Work out the finished part from the listing and answer in its coordinate system (mm). A direction names the side the tool comes from. Give positions to 0.01 mm unless a question says otherwise; leave off trailing zeros. Order: outer loops, then holes, each group sorted by start corner. A loop starts at its lowest first (then second) coordinate and runs counter-clockwise, first axis right, second up. Notation, with made-up numbers: (-31.5, 15) - (26.5, 15) arc R23 ccw to (26.5, 27) - close; hole circle Ø1 at (-12, 45.25). An arc over 180 degrees is marked (long way). Put each result on its own line as item: value.
```python
from build123d import *

# Parameters (mm, degrees)
F1_DEPTH = 25.4


with BuildPart() as f1:
    # F0 (on Front) → F1 (new body)
    with BuildSketch(Plane.XZ):
        with BuildLine():
            Line((5.7565809201, 24.7419614515), (-18.5488766964, 17.3563260415))
            Line((-18.5488766964, 17.3563260415), (-24.3054576165, -7.38563541))
            Line((-24.3054576165, -7.38563541), (-5.7565809201, -24.7419614515))
            Line((-5.7565809201, -24.7419614515), (18.5488766964, -17.3563260415))
            Line((18.5488766964, -17.3563260415), (9.9212024357, -6.0961798708))
            ThreePointArc((9.9212024357, -6.0961798708), (-11.27855426, -2.8961837982), (5.7565809201, 10.1220276081))
            Line((5.7565809201, 10.1220276081), (5.7565809201, 24.7419614515))
        make_face()
        with BuildLine():
            ThreePointArc((11.6444693648, 0), (10.0654358316, 5.8549695395), (5.7565809201, 10.1220276081))
            Line((5.7565809201, 10.1220276081), (5.7565809201, -0.6608509982))
            Line((5.7565809201, -0.6608509982), (9.9212024357, -6.0961798708))
            ThreePointArc((9.9212024357, -6.0961798708), (11.2053738138, -3.1675328698), (11.6444693648, 0))
        make_face()
        with BuildLine():
            Line((5.7565809201, -0.6608509982), (5.7565809201, 10.1220276081))
            ThreePointArc((5.7565809201, 10.1220276081), (-11.27855426, -2.8961837982), (9.9212024357, -6.0961798708))
            Line((9.9212024357, -6.0961798708), (5.7565809201, -0.6608509982))
        make_face()
    extrude(amount=F1_DEPTH)


solid = f1.part
```
(1) Given pin 1 (10 mm diameter, centred on y = -19.5, z = -19.5, fed in from -X); pin 2 (10 mm diameter, centred on x = -10.5, y = -21.5, fed in from +Z); pin 3 (2 mm diameter, centred on x = -3.5, y = -21, fed in from +Z), each flat-ended and moving along its own axis, determine where each tip first touches the part or whether it passes through.
Geometry check:
pin 1: stops at x = -16.7
pin 2: stops at z = 21.32
pin 3: stops at z = 22.23
(2) A tool of negligible diameter and unlimited length cuts with its end or side. For faces 1 (the face through (-21.387, -12.522, 5.159)), 2 (the face through (5.757, -13, 17)), from which of +Z, -Z, +X, -X, +Y, -Y can it reach the whole face along a straight path? Write none if from no direction.
Geometry check:
face 1: +Z, -X, +Y, -Y
face 2: +Z, +X, +Y, -Y
(3) Straight lines are drawn through the part: line 1 (Z direction, x = -15.5, y = -10); line 2 (Z direction, x = -10, y = -13.25); line 3 (X direction, y = -4.5, z = 13). For each, find the intervals that lie inside material, in ascending order.
Geometry check:
line 1: z = -15.62 to 18.28
line 2: z = -20.77 to 19.95
line 3: x = -19.56 to 5.76
(4) Determine the mould class of faces 3 (the face through (14.3, -12.52, -11.81)), 4 (the face through (-3, 0, 0)), 5 (the face through (-6.23, -12.52, 21.1)) for opening direction Z: pulls with the +Z half, pulls with the -Z half, needs draft (parallel to the pull), parting line crosses it, or undercut.
Geometry check:
face 3: undercut
face 4: needs draft
face 5: pulls with the +Z half
(5) Section C-C, the plane x = 13 is taken. Write down the section's boundary in (y, z).
Geometry check:
outline: (-25.4, -19.04) - (0, -19.04) - (0, -10.11) - (-25.4, -10.11) - close
(6) Section A-A, the plane y = -6 is taken. Write down the section's boundary in (x, z).
Geometry check:
outline: (-24.31, -7.39) - (-5.76, -24.74) - (18.55, -17.36) - (9.92, -6.1) arc R11.64 ccw to (5.76, 10.12) - (5.76, 24.74) - (-18.55, 17.36) - close
(7) Section B-B, the plane z = -21 is taken. Write down the section's boundary in (x, y).
Geometry check:
outline: (-9.76, -25.4) - (6.56, -25.4) - (6.56, 0) - (-9.76, 0) - close
